Design review of the part shown in the three views and the two pictorial views. Dimensions are in mm from the part's minimum x, y and z. Round coordinates to 2 decimals unless told otherwise and drop trailing zeros. Loops run counter-clockwise (first coordinate to the right, second up) from the corner with the lowest first, then second, coordinate; pieces in that order, holes last. Notation, with made-up numbers: (89, -19.75) -> (121, -19.75) arc R13 ccw to (121, -8.75) -> close; hole circle Ø2 at (61.25, 35.25). An arc over 180 degrees is marked (long way). One line per question, with ' | ' between items. Start each with the question number.
1. Consider section A-A (y = 0.7). Write out the cut boundary in (x, z), and give its area (3 significant figures).
2. For pin 1 Ø3 at (x, z) = (6.35, 63.5) entering from -Y; pin 2 Ø1.5 at (y, z) = (2, 35) entering from -X, all flat-tipped, find the tip position at first contact; note any pin that passes through.
3. Consider section B-B (z = 8). Write out the cut boundary in (x, y).
4. Wall thickness on line 1 along X through (y, z) = (2.2, 6.35); line 2 along X through (y, z) = (0.3, 64): over which ranges is each line inside the solid? List them lowest first.
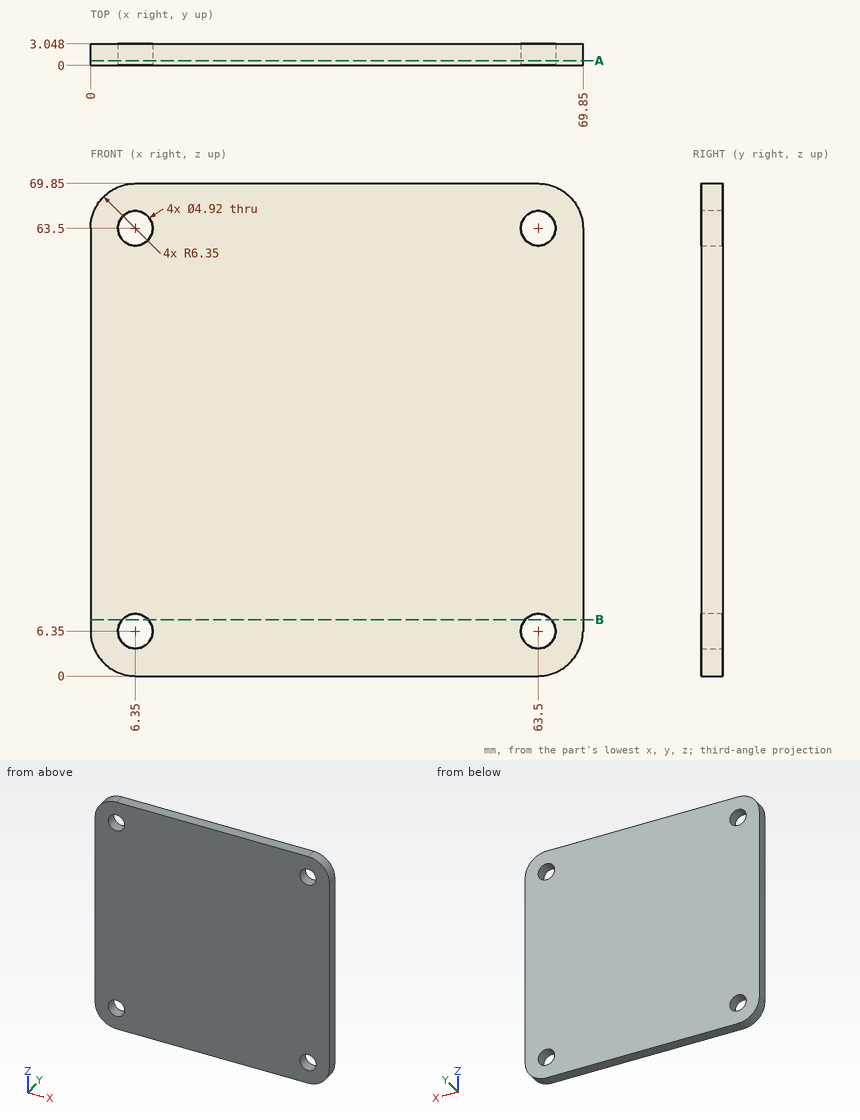
Answer block:
1) outline: (0, 6.35) arc R6.35 ccw to (6.35, 0) -> (63.5, 0) arc R6.35 ccw to (69.85, 6.35) -> (69.85, 63.5) arc R6.35 ccw to (63.5, 69.85) -> (6.35, 69.85) arc R6.35 ccw to (0, 63.5) -> close; hole circle Ø4.92 at (6.35, 6.35); hole circle Ø4.92 at (6.35, 63.5); hole circle Ø4.92 at (63.5, 6.35); hole circle Ø4.92 at (63.5, 63.5) | area: 4,770 mm2
2) pin 1: passes through | pin 2: stops at x = 0
3) outline: (0, 0) -> (4.53, 0) -> (4.53, 3.05) -> (0, 3.05) -> close; (8.17, 0) -> (61.68, 0) -> (61.68, 3.05) -> (8.17, 3.05) -> close; (65.32, 0) -> (69.85, 0) -> (69.85, 3.05) -> (65.32, 3.05) -> close
4) line 1: x = 0 to 3.89, 8.81 to 61.04, 65.96 to 69.85 | line 2: x = 0.02 to 3.94, 8.76 to 61.09, 65.91 to 69.83
